Read the model definition and answer for the solid it produces. Units are mm, in the model's axes. Coordinates: 2 decimals unless noted, no trailing zeros. Write each loop counter-clockwise with the first axis right and the second up, starting at its lowest first coordinate (ties: lowest second). Pieces come first, ordered by that corner, then holes. Notation, with made-up numbers: (52.25, 87) -> (102.25, 87) arc R37 ccw to (102.25, 124) -> close; hole circle Ø4 at (57.5, -11.75). An arc over 180 degrees is marked (long way). Answer in a Markdown table with one row per item. Add a question column.
Item 1: Section C-C on x = 0 is taken. Write down the section's boundary in (y, z).
Item 2: Section A-A on z = 0 is taken. Write down the section's boundary in (x, y).
Item 3: Given pin 1 Ø2 at (y, z) = (2.5, 26) entering from +X; pin 2 Ø4 at (x, y) = (10, 2) entering from +Z; pin 3 Ø1.5 at (y, z) = (5.5, 12.5) entering from +X; pin 4 Ø4.5 at (x, y) = (0, 3.17) entering from +Z, each flat-ended and moving along its own axis, determine where each tip first touches the part or whether it passes through.
Item 4: Section B-B on x = -29.5 is taken. Write down the section's boundary in (y, z), then the cut area to 3 significant figures.
Item 5: Section D-D on y = 5.75 is taken. Write down the section's boundary in (x, z), then the cut area to 3 significant figures.
Item 6: Straight lines are drawn through the part: line 1 (Y direction, x = 0, z = 37.15); line 2 (X direction, y = 4, z = 0); line 3 (Z direction, x = 10, y = 2.25). For each, find the intervals that lie inside material, in ascending order. Write a range as from..to.
Item 7: For a pull along Y with two mould halves and no side action, classify faces 1 (the face through (35.123, 2.027, 11.456)), 2 (the face through (28, 7.62, 23)), 3 (the face through (28, 0, 23)) as +Y half, -Y half, draft (parallel to the pull), parting line (faces both ways), or undercut.
```python
from build123d import *

# Parameters (mm, degrees)
SKETCH1_R                       = 37.973
SKETCH1_R_2                     = 35.941
BOSS_EXTRUDE1_DEPTH             = 7.62
SKETCH2_R                       = 1.692869147
CUT_EXTRUDE1_DEPTH              = 86.62
CIRPATTERN1_COUNT               = 2
CIRPATTERN2_COUNT               = 2
CIRPATTERN2_ANGLE               = 70
CIRPATTERN2_THE_OTHER_WAY_COUNT = 2
CIRPATTERN2_THE_OTHER_WAY_ANGLE = 70


with BuildPart() as part:
    # Sketch1 → Boss-Extrude1 (new body)
    with BuildSketch(Plane(origin=(0, 0, 0), x_dir=(1, 0, 0), z_dir=(0, 1, 0))):
        with Locations(Location((0, 0, 0), (0, 0, 90))):
            Circle(SKETCH1_R)
        with Locations(Location((0, 0, 0), (0, 0, 90))):
            Circle(SKETCH1_R_2, mode=Mode.SUBTRACT)
    extrude(amount=BOSS_EXTRUDE1_DEPTH)

    # Sketch2 → Cut-Extrude1 (cut)
    with BuildSketch(Plane.XY):
        with Locations(Location((0, 3.171011831, 0), (0, 0, 180))):
            Circle(SKETCH2_R)
    cut_extrude1 = extrude(amount=CUT_EXTRUDE1_DEPTH, mode=Mode.SUBTRACT)

    # CirPattern1: Cut-Extrude1 ×2 about axis
    cirpattern1_axis = Axis((0, 7.62, 0), (0, -1, 0))
    for i in range(1, CIRPATTERN1_COUNT):
        add(cut_extrude1.rotate(cirpattern1_axis, i * 360 / CIRPATTERN1_COUNT), mode=Mode.SUBTRACT)

    # CirPattern2: Cut-Extrude1 ×2 about axis
    cirpattern2_axis = Axis((0, 7.62, 0), (0, 1, 0))
    for i in range(1, CIRPATTERN2_COUNT):
        add(cut_extrude1.rotate(cirpattern2_axis, i * CIRPATTERN2_ANGLE / (CIRPATTERN2_COUNT - 1)), mode=Mode.SUBTRACT)

    # CirPattern2 the other way: Cut-Extrude1 ×2 about axis
    cirpattern2_the_other_way_axis = Axis((0, 7.62, 0), (0, -1, 0))
    for i in range(1, CIRPATTERN2_THE_OTHER_WAY_COUNT):
        add(cut_extrude1.rotate(cirpattern2_the_other_way_axis, i * CIRPATTERN2_THE_OTHER_WAY_ANGLE / (CIRPATTERN2_THE_OTHER_WAY_COUNT - 1)), mode=Mode.SUBTRACT)


solid = part.part
```
Results below:
| question | item | result |
|---|---|---|
| 1 | outline | (0, -37.97) -> (1.48, -37.97) -> (1.48, -35.94) -> (0, -35.94) -> close; (0, 35.94) -> (1.48, 35.94) -> (1.48, 37.97) -> (0, 37.97) -> close; (4.86, -37.97) -> (7.62, -37.97) -> (7.62, -35.94) -> (4.86, -35.94) -> close; (4.86, 35.94) -> (7.62, 35.94) -> (7.62, 37.97) -> (4.86, 37.97) -> close |
| 2 | outline | (-37.97, 0) -> (-35.94, 0) -> (-35.94, 7.62) -> (-37.97, 7.62) -> close; (35.94, 0) -> (37.97, 0) -> (37.97, 7.62) -> (35.94, 7.62) -> close |
| 3 | pin 1 | stops at x = 28.58 |
| 3 | pin 2 | stops at z = 37.12 |
| 3 | pin 3 | stops at x = 36.11 |
| 3 | pin 4 | stops at z = 37.97 |
| 4 | outline | (0, -23.91) -> (7.62, -23.91) -> (7.62, -20.53) -> (0, -20.53) -> close; (0, 20.53) -> (7.62, 20.53) -> (7.62, 23.91) -> (0, 23.91) -> close |
| 4 | area | 51.5 mm2 |
| 5 | outline | circle Ø75.95 at (0, 0); hole circle Ø71.88 at (0, 0) |
| 5 | area | 472 mm2 |
| 6 | line 1 | y = 0..1.48, 4.86..7.62 |
| 6 | line 2 | x = -37.97..-35.94, 35.94..37.97 |
| 6 | line 3 | z = -36.63..-34.52, 34.52..36.63 |
| 7 | face 1 | undercut |
| 7 | face 2 | +Y half |
| 7 | face 3 | -Y half |
